Read the model definition and answer for the solid it produces. Units are mm, in the model's axes. A direction names the side the tool comes from. Coordinates: 2 decimals unless noted, no trailing zeros. Write each loop counter-clockwise with the first axis right and the second up, starting at its lowest first coordinate (ties: lowest second). Pieces come first, ordered by that corner, then holes. Notation, with made-up numbers: (-16, -34.75) -> (26, -34.75) arc R35 cw to (26, 1.25) -> close; hole circle Ø6 at (20, 53.5). An arc over 180 degrees is marked (long way). Write item = value, one per line. Start each with the question number.
1) For a pull along Y with two mould halves and no side action, classify faces 1 (the face through (-6.43, -20.4, 0.74)), 2 (the face through (-6.342, -7.454, 0.74)), 3 (the face through (7.642, -9, 1)), 4 (the face through (-8.79, -6.48, 0.74)) as released by +Y, released by -Y, zero draft, split by the parting line, or undercut.
2) Section B-B (x = -1.5) is taken. Determine the outline of the cut face in (y, z) (3 decimals), plus the area to 3 significant figures.
3) Find the intervals of material crossed by line 1 along Y through (x, z) = (4.25, 0.15) (3 decimals); line 2 along Y through (x, z) = (-7, 1.15) (3 decimals); line 3 along Y through (x, z) = (-8, 0.85), in increasing order. Write a range as from..to.
4) Section A-A (y = -25.25) is taken. Determine the outline of the cut face in (x, z).
5) Section C-C (z = 1.25) is taken. Count the separate pieces of the cut face and the enclosed holes in it, plus the area to 3 significant figures.
6) Section D-D (y = -20.25) is taken. Determine the outline of the cut face in (x, z).
7) Flat-ended cylindrical pins translate along their axes: pin 1 Ø1.3 at (x, y) = (-1.36, -21.88) entering from +Z; pin 2 Ø0.8 at (x, z) = (-2.5, 0.5) entering from -Y. Find the tip coordinate at first contact, or state that the pin passes through.
8) A tool of negligible diameter and unlimited length cuts with its end or side. For faces 5 (the face through (4.16, -20.66, 0.74)), 6 (the face through (-9.358, -18, 1)), from which of +Z, -Z, +X, -X, +Y, -Y can it reach the whole face along a straight path? Write none if from no direction.
Autodesk Inventor part; units mm, degrees
ref_plane "YZ Plane" through (0, 0, 0) normal (1, 0, 0) x (0, 1, 0)
ref_plane "XZ Plane" through (0, 0, 0) normal (0, 1, 0) x (-1, 0, 0)
ref_plane "XY Plane" through (0, 0, 0) normal (0, 0, 1) x (1, 0, 0)
sketch "スケッチ1" plane through (0, 0, 0) normal (0, 0, 1) x (1, 0, 0)
  circle A0 centre (5.6422, -7.875) radius 1
  circle A1 centre (-7.3578, -7.875) radius 1
  circle A2 centre (5.6422, -7.875) radius 1.1
  circle A3 centre (-7.3578, -7.875) radius 1.1
  circle A4 centre (-1.3578, -27.875) radius 4.1
  circle A5 centre (-1.3578, -27.875) radius 4
  circle A6 centre (4.6422, -27.875) radius 1.1
  circle A7 centre (-1.3578, -27.875) radius 6 construction
  circle A8 centre (2.8849, -23.6324) radius 1.1
  circle A9 centre (-1.3578, -21.875) radius 1.1
  circle A10 centre (-5.6004, -23.6324) radius 1.1
  circle A11 centre (-7.3578, -27.875) radius 1.1
  circle A12 centre (-5.6004, -32.1176) radius 1.1
  circle A13 centre (-1.3578, -33.875) radius 1.1
  circle A14 centre (2.8849, -32.1176) radius 1.1
  line L0 (7.6422, -5.875) -> (-9.3578, -5.875)
  line L1 (-9.3578, -5.875) -> (-9.3578, -9.875)
  line L2 (-9.3578, -9.875) -> (7.6422, -9.875)
  line L3 (7.6422, -9.875) -> (7.6422, -5.875)
  circle A15 centre (-1.3578, -27.875) radius 8
  line L4 (6.6302, -28.3134) -> (7.6422, -9.875)
  line L5 (-9.3578, -27.875) -> (-9.3578, -9.875)
  circle A16 centre (5.6422, -7.875) radius 2
  circle A17 centre (-7.3578, -7.875) radius 2
  point P0 (0, 0)
  point P1 (5.6422, -5.875)
  point P2 (-7.3578, -5.875)
  point P3 (-9.3578, -7.875)
  point P4 (7.6422, -7.875)
  dimension "d4" = 12
  dimension "d0" = 2.2
  dimension "d1" = 2.2
  dimension "d2" = 8
  dimension "d3" = 2.2
  dimension "d7" = 360
  dimension "d9" = 16
  dimension "d10" = 4
  dimension "d11" = 4
extrude "押し出し1" add sketch "スケッチ1" along normal blind 1.5 contours A4 | A16 L2 A17 L0 | A16 | L3 L2 A16 | A17 | L2 L4 A15 L5 | A17 L2 L1 | A15
sketch "スケッチ2" plane through (0, 0, 1.5) normal (0, 0, 1) x (1, 0, 0)
  arc A0 (-7.3578, -5.875) -> (-9.3578, -7.875) centre (-7.3578, -7.875) ccw
  line L0 (-9.3578, -7.875) -> (-9.3578, -27.875)
  arc A1 (-9.3578, -27.875) -> (6.6302, -28.3134) centre (-1.3578, -27.875) ccw
  line L1 (6.6302, -28.3134) -> (7.6422, -9.875)
  line L2 (7.6422, -9.875) -> (7.6422, -7.875)
  arc A2 (7.6422, -7.875) -> (5.6422, -5.875) centre (5.6422, -7.875) ccw
  line L3 (5.6422, -5.875) -> (-7.3578, -5.875)
  circle A3 centre (4.6422, -27.875) radius 1.1
  circle A4 centre (2.8849, -23.6324) radius 1.1
  circle A5 centre (-1.3578, -21.875) radius 1.1
  circle A6 centre (-5.6004, -23.6324) radius 1.1
  circle A7 centre (-7.3578, -27.875) radius 1.1
  circle A8 centre (-5.6004, -32.1176) radius 1.1
  circle A9 centre (-1.3578, -33.875) radius 1.1
  circle A10 centre (2.8849, -32.1176) radius 1.1
  circle A11 centre (-1.3578, -27.875) radius 4
  circle A12 centre (5.6422, -7.875) radius 1.1
  circle A13 centre (-7.3578, -7.875) radius 1.1
  line L4 (5.6422, -9.8202) -> (4.6332, -28.2038)
  arc A14 (-7.3578, -27.875) -> (4.6332, -28.2038) centre (-1.3578, -27.875) ccw
  line L5 (-7.3578, -27.875) -> (-7.3578, -7.875)
  line L6 (-7.3578, -7.875) -> (5.6422, -7.875)
  line L7 (5.6422, -7.875) -> (5.6422, -9.8202)
  circle A15 centre (5.6422, -7.875) radius 2
  circle A16 centre (-7.3578, -7.875) radius 2
  circle A17 centre (-1.3578, -27.875) radius 8
  point P0 (0, 0)
  point P1 (-7.3578, -22.5835)
  point P2 (4.9232, -22.9203)
  point P3 (5.6392, -9.875)
  point P4 (3.6422, -7.875)
  point P5 (-5.3578, -7.875)
  point P6 (-7.3578, -9.875)
  dimension "d14" = 2
  dimension "d15" = 16
extrude "押し出し2" cut sketch "スケッチ2" against normal through all contours L6 A15 L4 A17 L5 A16
fillet "フィレット1" radius 2 6 edges at (4.9232, -22.9203, 0.75) (-7.3578, -22.5835, 0.75) (-7.3578, -9.875, 0.75) (-5.3578, -7.875, 0.75) (5.6392, -9.875, 0.75) (3.6422, -7.875, 0.75)
properties part number "newnewude_2" material "アルミニウム 2014-T4"
Answer key:
q1.face_1 = undercut
q1.face_2 = undercut
q1.face_3 = zero draft
q1.face_4 = released by +Y
q2.outline = (-35.874, 0) -> (-34.966, 0) -> (-34.966, 1.5) -> (-35.874, 1.5) -> close; (-32.784, 0) -> (-31.872, 0) -> (-31.872, 1.5) -> (-32.784, 1.5) -> close; (-23.878, 0) -> (-22.966, 0) -> (-22.966, 1.5) -> (-23.878, 1.5) -> close; (-20.784, 0) -> (-19.876, 0) -> (-19.876, 1.5) -> (-20.784, 1.5) -> close; (-7.875, 0) -> (-5.875, 0) -> (-5.875, 1.5) -> (-7.875, 1.5) -> close
q2.area = 8.46 mm^2
q3.line_1 = -33.58..-28.903, -26.847..-20.606, -9.311..-5.875
q3.line_2 = -33.546..-28.915, -26.835..-19.851, -10.198..-8.915, -6.835..-5.875
q3.line_3 = -32.33..-28.77, -26.98..-8.77, -6.98..-5.98
q4.outline = (-9.36, 0) -> (-4.38, 0) -> (-4.38, 1.5) -> (-9.36, 1.5) -> close; (1.66, 0) -> (6.8, 0) -> (6.8, 1.5) -> (1.66, 1.5) -> close
q5.separate_pieces = 1
q5.enclosed_holes = 12
q5.area = 225 mm^2
q6.outline = (-9.36, 0) -> (-6.63, 0) -> (-6.63, 1.5) -> (-9.36, 1.5) -> close; (-3.78, 0) -> (1.06, 0) -> (1.06, 1.5) -> (-3.78, 1.5) -> close; (4.65, 0) -> (7.07, 0) -> (7.07, 1.5) -> (4.65, 1.5) -> close
q7.pin_1 = through
q7.pin_2 = -35.84
q8.face_5 = +Z, -Z
q8.face_6 = +Z, -Z, -X, +Y, -Y
